The listing builds one solid part. Answer for the finished solid, in the listing's coordinates (mm). A direction names the side the tool comes from. Coordinates: 2 decimals unless noted, no trailing zeros. Write each loop counter-clockwise with the first axis right and the second up, starting at its lowest first coordinate (ties: lowest second). Pieces come first, ordered by that corner, then holes.
```python
from build123d import *

# Parameters (mm, degrees)
SKETCH1_W           = 59.69
SKETCH1_H           = 24.384
BOSS_EXTRUDE2_DEPTH = 3.175
SKETCH3_W           = 11.938
SKETCH3_H           = 3.175
CUT_EXTRUDE2_DEPTH  = 3.175
LPATTERN2_COUNT     = 2
LPATTERN2_PITCH     = 23.876
SKETCH4_W           = 6.35
SKETCH4_H           = 8.128
CUT_EXTRUDE3_DEPTH  = 3.175
SKETCH5_W           = 9.525
SKETCH5_H           = 11.303
SKETCH5_W_2         = 12.5095
SKETCH5_H_2         = 11.43
CUT_EXTRUDE4_DEPTH  = 3.175


with BuildPart() as part:
    # Sketch1 → Boss-Extrude2 (new body)
    with BuildSketch(Plane(origin=(0, 0, 0), x_dir=(1, 0, 0), z_dir=(0, 1, 0))):
        Rectangle(SKETCH1_W, SKETCH1_H)
    extrude(amount=BOSS_EXTRUDE2_DEPTH)

    # Sketch3 → Cut-Extrude2 (cut)
    with BuildSketch(Plane(origin=(0, 3.175, 0), x_dir=(1, 0, 0), z_dir=(0, 1, 0))):
        with Locations((11.938, 10.6045)):
            Rectangle(SKETCH3_W, SKETCH3_H)
        with Locations((11.938, -10.6045)):
            Rectangle(SKETCH3_W, SKETCH3_H)
    cut_extrude2 = extrude(amount=-CUT_EXTRUDE2_DEPTH, mode=Mode.SUBTRACT)

    # LPattern2: Cut-Extrude2 ×2
    with Locations(*[(-i * LPATTERN2_PITCH, 0, 0) for i in range(1, LPATTERN2_COUNT)]):
        add(cut_extrude2, mode=Mode.SUBTRACT)

    # Sketch4 → Cut-Extrude3 (cut)
    with BuildSketch(Plane(origin=(0, 3.175, 0), x_dir=(1, 0, 0), z_dir=(0, 1, 0))):
        with Locations((-29.845, 0)):
            Rectangle(SKETCH4_W, SKETCH4_H)
        with Locations((29.845, 0)):
            Rectangle(SKETCH4_W, SKETCH4_H)
    extrude(amount=-CUT_EXTRUDE3_DEPTH, mode=Mode.SUBTRACT)

    # Sketch5 → Cut-Extrude4 (cut)
    with BuildSketch(Plane(origin=(0, 3.175, 0), x_dir=(1, 0, 0), z_dir=(0, 1, 0))):
        with Locations((-19.1135, -0.1905)):
            Rectangle(SKETCH5_W, SKETCH5_H)
        with Locations((10.89025, -0.127)):
            Rectangle(SKETCH5_W_2, SKETCH5_H_2)
    extrude(amount=-CUT_EXTRUDE4_DEPTH, mode=Mode.SUBTRACT)


solid = part.part
```
(1) Section D-D, the plane z = 10.5 is taken. Write down the section's boundary in (x, y) (3 decimals), plus the area to 3 significant figures.
(2) Section B-B, the plane x = -17 is taken. Write down the section's boundary in (y, z) (3 decimals), plus the area to 3 significant figures.
(3) Section A-A, the plane z = 4.75 is taken. Write down the section's boundary in (x, y) (1 decimal).
(4) For a pull along Z with two mould halves and no side action, classify faces 4 (the flat face through (17.907, 2, 11)), 5 (the flat face through (17.145, 2, 0)), 6 (the flat face through (-24, 2, -12.192)) as pulls with the +Z half, pulls with the -Z half, needs draft (parallel to the pull), parting line crosses it, or undercut.
(5) Find the intervals of material crossed by probe 1 along X at (y, z) = (2.4, 0.75) (1 decimal); probe 2 along X at (y, z) = (2.6, 4.25) (1 decimal); probe 3 along Z at (x, y) = (12, 1.2), in increasing order.
(6) Section C-C, the plane x = 8 is taken. Write down the section's boundary in (y, z) (3 decimals).
(7) Which of the six approach directions +Z, -Z, +X, -X, +Y, -Y give full straight-line access (tool end or side, diameter ignored) to faces 1 (the flat face through (-14.351, 2, 0)), 2 (the flat face through (-28, 2, 4.064)), 3 (the flat face through (-12, 2, 9.017))?
(8) Each of these flat-tipped pins is pushed along its axis until it touches: pin 1 (1 mm diameter, centred on x = -13.5, y = 2, fed in from -Z); pin 2 (1 mm diameter, centred on x = 12, y = 2.5, fed in from +Z); pin 3 (1 mm diameter, centred on y = 2, z = -1, fed in from -X). Where does it stop, or does it pass through?
Solution:
1. outline: (-29.845, 0) - (-17.907, 0) - (-17.907, 3.175) - (-29.845, 3.175) - close; (-5.969, 0) - (5.969, 0) - (5.969, 3.175) - (-5.969, 3.175) - close; (17.907, 0) - (29.845, 0) - (29.845, 3.175) - (17.907, 3.175) - close
1. area: 114 mm2
2. outline: (0, -9.017) - (3.175, -9.017) - (3.175, -5.461) - (0, -5.461) - close; (0, 5.842) - (3.175, 5.842) - (3.175, 9.017) - (0, 9.017) - close
2. area: 21.4 mm2
3. outline: (-29.8, 0) - (-23.9, 0) - (-23.9, 3.2) - (-29.8, 3.2) - close; (-14.4, 0) - (4.6, 0) - (4.6, 3.2) - (-14.4, 3.2) - close; (17.1, 0) - (29.8, 0) - (29.8, 3.2) - (17.1, 3.2) - close
4. face 4: needs draft
4. face 5: undercut
4. face 6: pulls with the -Z half
5. probe 1: x = -26.7 to -23.9, -14.4 to 4.6, 17.1 to 26.7
5. probe 2: x = -29.8 to -23.9, -14.4 to 4.6, 17.1 to 29.8
5. probe 3: z = -9.02 to -5.59, 5.84 to 9.02
6. outline: (0, -9.017) - (3.175, -9.017) - (3.175, -5.588) - (0, -5.588) - close; (0, 5.842) - (3.175, 5.842) - (3.175, 9.017) - (0, 9.017) - close
7. face 1: +Y, -Y
7. face 2: -X, +Y, -Y
7. face 3: +Z, +Y, -Y
8. pin 1: stops at z = -9.02
8. pin 2: stops at z = 9.02
8. pin 3: stops at x = -26.67
